Autodesk Inventor part; units mm, degrees
ref_plane "Work Plane1" through (-23.7962, 0, 0) normal (0, -0.866, -0.5) x (1, 0, 0)
ref_plane "YZ Plane" through (0, 0, 0) normal (1, 0, 0) x (0, 1, 0)
ref_plane "XZ Plane" through (0, 0, 0) normal (0, 1, 0) x (-1, 0, 0)
sketch "Sketch1" plane through (0, 0, 0) normal (1, 0, 0) x (0, 1, 0)
  line L0 (-12.8316, 0) -> (-6.4158, 11.1125)
  line L1 (-6.4158, 11.1125) -> (6.4158, 11.1125)
  line L2 (6.4158, 11.1125) -> (12.8316, 0)
  line L3 (12.8316, 0) -> (6.4158, -11.1125)
  line L4 (6.4158, -11.1125) -> (-6.4158, -11.1125)
  line L5 (-6.4158, -11.1125) -> (-12.8316, 0)
  point P0 (0, 0)
  point P1 (0, 0)
  dimension "d0" = 25.6632
extrude "Body" add sketch "Sketch1" along normal blind 12.319
sketch "Sketch2" plane through (0, 0, 0) normal (0, 0, 1) x (1, 0, 0)
  line L0 (0, 6.4158) -> (0, 12.8316)
  line L1 (0, 12.8316) -> (12.319, 12.8316)
  line L2 (12.319, 6.4158) -> (12.319, 12.8316)
  line L3 (-2.4638, 0) -> (14.7828, 0)
  line L4 (0.9925, 12.8316) -> (0, 11.1125)
  line L5 (11.3265, 12.8316) -> (12.319, 11.1125)
  dimension "d3" = 30
  dimension "d4" = 30
  dimension "d5" = 22.225
  dimension "d6" = 22.225
revolve "Chamfer1" cut sketch "Sketch2" angle 360 about axis through (-10, 0, 0) along (1, 0, 0)
sketch "Sketch3" plane through (12.319, 0, 0) normal (1, 0, 0) x (0, 0, -1)
  arc A0 (-5.5562, -9.6237) -> (5.5563, -9.6237) centre (0, 0) ccw
hole "Thread" at (12.319, 0, 0) direction (-1, 0, 0) diameter 11.9888 end through all
chamfer "Chamfer2" distance 1.1457 angle 30 1 edges at (12.319, 0, 5.9944) measured on face at (12.319, -9.3513, -0.2408)
chamfer "Chamfer3" distance 1.1457 angle 30 1 edges at (0, 0, 5.9944) measured on face at (0, -9.3513, -0.2408)
ref_plane "Work Plane1" through (-23.7962, 0, 0) normal (0, -0.866, -0.5) x (1, 0, 0)
equation "\"d0\" = 1.1547 * SW"
equation "\"d1\" = KOH"
equation "\"d3\" = ANG1"
equation "\"d4\" = ANG2"
equation "\"d5\" = SW0"
equation "\"d6\" = SW01"
equation "\"d8\" = -0.5 * GD1 + 0.5 * NND"
equation "\"d40\" = -0.5 * GD1 + 0.5 * NND"
equation "\"d10\" = -0.5 * GD1 + 0.5 * NND"
equation "\"d41\" = -0.5 * GD1 + 0.5 * NND"
equation "\"ANG1\" = 30deg"
equation "\"ANG2\" = 30deg"
equation "\"NND\" = 14.2875"
equation "\"KOH\" = 12.319"
equation "\"SW\" = 22.225"
equation "\"SW0\" = SW"
equation "\"SW01\" = SW"
equation "\"THREADDIA\" = 14.2875"
equation "\"TOA\" = 30deg"
equation "\"E0\" = 1.155 * SW"
properties part number "ANSI B18.2.2 - 9/16 - 12, HNI" material "Steel, Mild"
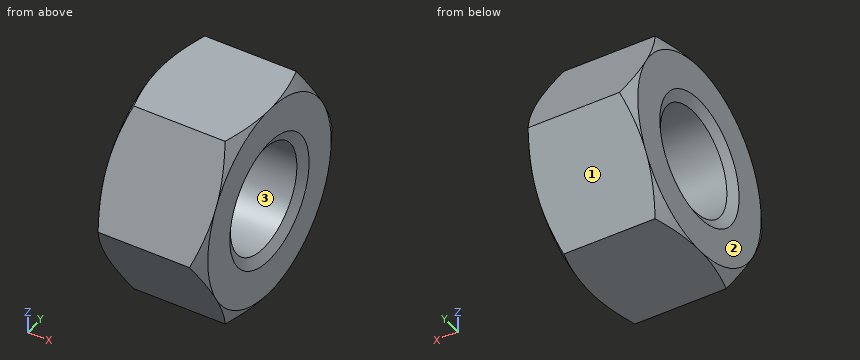
Design review of the part built by this model. Coordinates are the model's own, in mm. Face numbers are marked on the shaded views. Give positions to 0.01 mm unless a question says otherwise; leave off trailing zeros. Write each loop counter-clockwise with the first axis right and the second up, starting at its lowest first coordinate (ties: lowest second). Pieces come first, ordered by that corner, then holes. Notation, with made-up numbers: (10.25, -28.75) -> (26.25, -28.75) arc R23 ccw to (26.25, 9.25) -> close; hole circle Ø2 at (-22, -2). An arc over 180 degrees is marked (long way). Answer in a Markdown table with one row per item.
(1) Consider section A-A (x = 4.5). State the section outline as (y, z) points.
Results:
| item | result |
|---|---|
| outline | (-12.83, 0) -> (-6.42, -11.11) -> (6.42, -11.11) -> (12.83, 0) -> (6.42, 11.11) -> (-6.42, 11.11) -> close; hole circle Ø11.99 at (0, 0) |
(2) To check wall thickness, follow probe 1 along Z at (x, y) = (4.5, 0); probe 2 along Y at (x, z) = (1.5, -1.25); probe 3 along Y at (x, z) = (7.75, -3.5). State the ranges of each line that lie inside material, in increasing order.
Results:
| item | result |
|---|---|
| probe 1 | -11.11 to -5.99, 5.99 to 11.11 |
| probe 2 | -12.11 to -5.86, 5.86 to 12.11 |
| probe 3 | -10.81 to -4.87, 4.87 to 10.81 |
(3) Clearance check with flat-ended pins moving along their axes: pin 1 (1 mm diameter, centred on y = 5, z = 4, fed in from +X); pin 2 (1 mm diameter, centred on x = 5.5, z = 5.5, fed in from -Y). State where each tip first meets the part, or that it passes through.
Results:
| item | result |
|---|---|
| pin 1 | x = 12.18 |
| pin 2 | y = -9.94 |
(4) Mouldability with a two-part tool opening along Y and no side actions: class the marked faces 1, 2 and 3 as +Y half, -Y half, draft (parallel to the pull), parting line (faces both ways), or undercut.
Results:
| item | result |
|---|---|
| face 1 | +Y half |
| face 2 | draft |
| face 3 | undercut |
